Solid Edge part; units mm, degrees
sketch "Sketch1" plane through (0, 0, 0) normal (1, 0, 0) x (0, 1, 0)
  line L0 (0, 65) -> (0, 27.25)
  line L1 (0, 27.25) -> (-20, 27.25)
  line L2 (-20, 27.25) -> (-20, 0)
  line L3 (-20, 0) -> (10, 0)
  line L4 (10, 0) -> (10, 65)
  line L5 (10, 65) -> (0, 65)
revolve "RevolvedProtrusion1" add sketch "Sketch1" angle 360 about axis through (0, -20, 0) along (0, 1, 0)
hole "Agujero_1" at (0, -20, 0) direction (0, 1, 0) diameter 20 end up to next counterbore diameter 30 counterbore depth 20
chamfer "Chaflán_1" distance 3 angle 45 1 edges at (0, -20, 27.25)
properties material "Acero ASTM A36"
Work out the finished part from the listing and answer in its coordinate system (mm). A direction names the side the tool comes from. Coordinates: 2 decimals unless noted, no trailing zeros. Loops run counter-clockwise (first coordinate to the right, second up) from the corner with the lowest first, then second, coordinate; pieces in that order, holes last. Notation, with made-up numbers: (87.5, 33.25) -> (114.5, 33.25) arc R26 cw to (114.5, 72.25) -> close; hole circle Ø5 at (77, 1.25). An arc over 180 degrees is marked (long way). Write each question's results on one line, items separated by ' | '. Start each with the question number.
1) Find section C-C on y = 8. Determine the outline of the cut face in (x, z), then the cut area to 3 significant figures.
2) Find section A-A on x = 0. Determine the outline of the cut face in (y, z), then the cut area to 3 significant figures.
3) The mould has two halves that part along X. Classify faces 3 (the conical face through (-21.68, -19.81, 11.28)), 4 (the cylindrical face through (-0.66, -9.86, 14.985)), 5 (the flat face through (1, 10, 14)): pulls with the +X half, pulls with the -X half, needs draft (parallel to the pull), parting line crosses it, or undercut.
4) Find section B-B on z = 0. Determine the outline of the cut face in (x, y).
5) For faces 1 (the flat face through (1, 0, 28)), 2 (the cylindrical face through (-9.76, 4.93, 2.17)), determine the directions among +Z, -Z, +X, -X, +Y, -Y from which every point of the face is accessible in a straight line to the end or side of a thin tool.
6) Flat-ended cylindrical pins translate along their axes: P1, Ø8, axis at y = -5, z = 6, coming from the -X side; P2, Ø1.5, axis at y = 3, z = -47, coming from the -X side; P3, Ø9, axis at x = -6, z = -4.5, coming from the -Y side. Find the tip coordinate at first contact, or state that the pin passes through.
7) Find section D-D on y = -12.75. Determine the outline of the cut face in (x, z), then the cut area to 3 significant figures.
8) Consider line 1 along X through (y, z) = (4, 0); line 2 along Y through (x, z) = (8, -52.5); line 3 along Z through (x, y) = (-13, -11.5). Determine where each line is inside the solid, lowest interval first.
Response values:
1) outline: circle Ø130 at (0, 0); hole circle Ø20 at (0, 0) | area: 13,000 mm^2
2) outline: (-20, -24.25) -> (-17, -27.25) -> (0, -27.25) -> (0, -65) -> (10, -65) -> (10, -10) -> (0, -10) -> (0, -15) -> (-20, -15) -> close; (-20, 15) -> (0, 15) -> (0, 10) -> (10, 10) -> (10, 65) -> (0, 65) -> (0, 27.25) -> (-17, 27.25) -> (-20, 24.25) -> close | area: 1,580 mm^2
3) face 3: parting line crosses it | face 4: undercut | face 5: needs draft
4) outline: (-65, 0) -> (-27.25, 0) -> (-27.25, -17) -> (-24.25, -20) -> (-15, -20) -> (-15, 0) -> (-10, 0) -> (-10, 10) -> (-65, 10) -> close; (10, 0) -> (15, 0) -> (15, -20) -> (24.25, -20) -> (27.25, -17) -> (27.25, 0) -> (65, 0) -> (65, 10) -> (10, 10) -> close
5) face 1: -Y | face 2: +Y, -Y
6) P1: stops at x = -27.18 | P2: stops at x = -45.67 | P3: stops at y = 0
7) outline: circle Ø54.5 at (0, 0); hole circle Ø30 at (0, 0) | area: 1,630 mm^2
8) line 1: x = -65 to -10, 10 to 65 | line 2: y = 0 to 10 | line 3: z = -23.95 to -7.48, 7.48 to 23.95
